Check sheet for the modelled part. Datum: model origin and axes. Units: mm. A direction names the side the tool comes from. Round coordinates to 2 decimals unless told otherwise and drop trailing zeros. Order: outer loops, then holes, each group sorted by start corner. A loop starts at its lowest first (then second) coordinate and runs counter-clockwise, first axis right, second up. Notation, with made-up numbers: (-6.5, -14.5) -> (14.5, -14.5) arc R15 cw to (14.5, -5.5) -> close; hole circle Ø9 at (-37.5, -26). An arc over 180 degrees is marked (long way). Answer in a Markdown table with one row per item.
```python
from build123d import *

# Parameters (mm, degrees)
SKETCH1_R           = 10
BOSS_EXTRUDE1_DEPTH = 10
SKETCH3_R           = 15
BOSS_EXTRUDE3_DEPTH = 10
SKETCH4_R           = 5
CUT_EXTRUDE1_DEPTH  = 20


with BuildPart() as part:
    # Sketch1 → Boss-Extrude1 (new body)
    with BuildSketch(Plane(origin=(0, 0, 0), x_dir=(0, 0, -1), z_dir=(1, 0, 0))):
        with BuildLine():
            ThreePointArc((16.967213115, -18.360655738), (0, 25), (-16.967213115, -18.360655738))
            ThreePointArc((-16.967213115, -18.360655738), (-7.5, -40), (-16.967213115, -61.639344262))
            ThreePointArc((-16.967213115, -61.639344262), (-24.653637732, -75.852935186), (-22.040471077, -91.799052281))
            ThreePointArc((-22.040471077, -91.799052281), (-7.5, -153.539335996), (-25.58571686, -214.33567452))
            ThreePointArc((-25.58571686, -214.33567452), (0, -260), (25.58571686, -214.33567452))
            ThreePointArc((25.58571686, -214.33567452), (7.5, -153.539335996), (22.040471077, -91.799052281))
            ThreePointArc((22.040471077, -91.799052281), (24.653637732, -75.852935186), (16.967213115, -61.639344262))
            ThreePointArc((16.967213115, -61.639344262), (7.5, -40), (16.967213115, -18.360655738))
        make_face()
        with Locations((0, -230)):
            Circle(SKETCH1_R, mode=Mode.SUBTRACT)
    extrude(amount=BOSS_EXTRUDE1_DEPTH)

    # Sketch3 → Boss-Extrude3 (add)
    with BuildSketch(Plane.ZY):
        Circle(SKETCH3_R)
        with Locations((0, -80)):
            Circle(SKETCH3_R)
    extrude(amount=BOSS_EXTRUDE3_DEPTH)

    # Sketch4 → Cut-Extrude1 (cut)
    with BuildSketch(Plane.ZY.offset(10)):
        with Locations((0, -80)):
            Circle(SKETCH4_R)
        Circle(SKETCH4_R)
    extrude(amount=-CUT_EXTRUDE1_DEPTH, mode=Mode.SUBTRACT)


solid = part.part
```
(1) Depth check by flat-ended pin: pin 1 Ø6 at (x, y) = (-4, -28.5) entering from -Z; pin 2 Ø18 at (y, z) = (-110, -5.5) entering from -X; pin 3 Ø10 at (x, y) = (0, -59) entering from +Z; pin 4 Ø1.5 at (x, z) = (6.5, 4.5) entering from -Y. Enter the tip coordinate at first touch or a pass-through.
Solutions:
| item | result |
|---|---|
| pin 1 | through |
| pin 2 | x = 0 |
| pin 3 | z = 19.21 |
| pin 4 | y = -259.76 |
(2) Section check D-D on y = -230. Record the boundary of the cut face in (x, z), plus the area to 3 significant figures.
Solutions:
| item | result |
|---|---|
| outline | (0, -30) -> (10, -30) -> (10, -10) -> (0, -10) -> close; (0, 10) -> (10, 10) -> (10, 30) -> (0, 30) -> close |
| area | 400 mm^2 |
(3) Scan lines: probe 1 along Y at (x, z) = (-5, 0); probe 2 along X at (y, z) = (-104.5, 8.5); probe 3 along Y at (x, z) = (-8, 2). Record each from-to range of solid material in increasing order. Write a range as from..to.
Solutions:
| item | result |
|---|---|
| probe 1 | -95..-85, -75..-65, -15..-5, 5..15 |
| probe 2 | 0..10 |
| probe 3 | -94.87..-84.58, -75.42..-65.13, -14.87..-4.58, 4.58..14.87 |
(4) Draft check along Z on faces 1 (the cylindrical face through (-4.93, -94.643, -3.252)), 2 (the cylindrical face through (-0.14, -4.88, -1.08)), 3 (the cylindrical face through (4.93, -152.642, 7.477)), 4 (the cylindrical face through (-0.14, -84.88, -1.08)). Enter one of: pulls with the +Z half, pulls with the -Z half, needs draft (parallel to the pull), parting line crosses it, or undercut.
Solutions:
| item | result |
|---|---|
| face 1 | parting line crosses it |
| face 2 | undercut |
| face 3 | pulls with the +Z half |
| face 4 | undercut |
(5) Section check B-B on y = -80. Record the boundary of the cut face in (x, z).
Solutions:
| item | result |
|---|---|
| outline | (-10, -15) -> (0, -15) -> (0, -25) -> (10, -25) -> (10, -5) -> (-10, -5) -> close; (-10, 5) -> (10, 5) -> (10, 25) -> (0, 25) -> (0, 15) -> (-10, 15) -> close |
(6) Section check A-A on z = 0. Record the boundary of the cut face in (x, y).
Solutions:
| item | result |
|---|---|
| outline | (-10, -95) -> (0, -95) -> (0, -220) -> (10, -220) -> (10, -85) -> (-10, -85) -> close; (-10, -75) -> (10, -75) -> (10, -5) -> (-10, -5) -> (-10, -15) -> (0, -15) -> (0, -65) -> (-10, -65) -> close; (-10, 5) -> (10, 5) -> (10, 25) -> (0, 25) -> (0, 15) -> (-10, 15) -> close; (0, -260) -> (10, -260) -> (10, -240) -> (0, -240) -> close |
(7) Tool access check on faces 5 (the cylindrical face through (4.93, -76.08, -24.69)), 6 (the cylindrical face through (-4.93, 0.66, -14.985)). Record the directions out of +Z, -Z, +X, -X, +Y, -Y that give a thin tool (end or side, any length) a straight path to the whole face; none if there is none.
Solutions:
| item | result |
|---|---|
| face 5 | -Z, +X, -X |
| face 6 | -X |
(8) Section check C-C on x = -7.5. Record the boundary of the cut face in (y, z).
Solutions:
| item | result |
|---|---|
| outline | circle Ø30 at (-80, 0); circle Ø30 at (0, 0); hole circle Ø10 at (-80, 0); hole circle Ø10 at (0, 0) |
